Could you check a few things on this model? Use its own coordinates, in mm. Face numbers are marked on the shaded views. A direction names the side the tool comes from. Coordinates: 2 decimals unless noted, no trailing zeros. Order: outer loops, then holes, each group sorted by start corner. A loop starts at its lowest first (then second) coordinate and runs counter-clockwise, first axis right, second up. Notation, with made-up numbers: (76, -31.5) -> (123, -31.5) arc R17 cw to (123, 0.5) -> close; hole circle Ø6 at (-9.75, -40). An arc over 180 degrees is marked (long way). Put each result on its own line as item: value. Start each with the question number.
Q1. For the marked faces 1 and 2, which set-ups out of +Z, -Z, +X, -X, +Y, -Y let a thin tool reach every point of the face, with its end or its side?
Q2. If we section it at A-A (z = 0): Please give me the cut outline in (x, y), and give its area (3 significant figures).
Q3. Please list where these lines run through material, in increasing order: line 1 along X through (y, z) = (3.75, 0); line 2 along Z through (x, y) = (0, 10).
Q4. We'd pull the mould along X, two halves only. Please class the marked faces 3, 4 and 5: +X half, -X half, draft (parallel to the pull), parting line (faces both ways), or undercut.
Q5. If we section it at B-B (y = 9.75): Please give me the cut outline in (x, z).
Q6. Will these pins go through, and if not, where does the flat tip stop? pin 1 (3 mm diameter, centred on y = 6, z = -3, fed in from +X); pin 2 (2 mm diameter, centred on x = -2.5, y = 10.5, fed in from -Z); pin 3 (5 mm diameter, centred on y = 11, z = -1, fed in from +X).
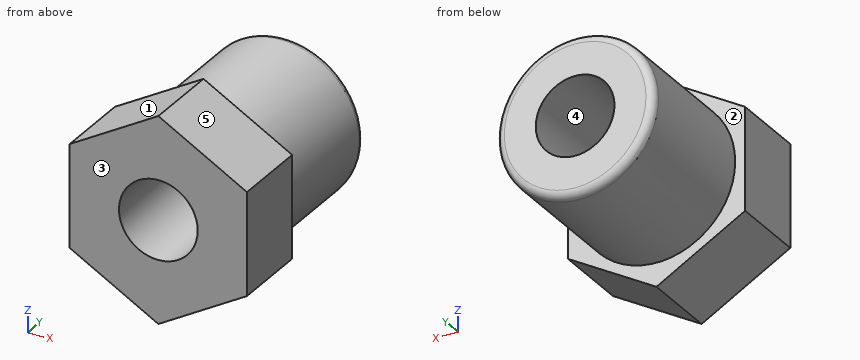
Autodesk Inventor part; units mm, degrees
ref_plane "YZ Plane" through (0, 0, 0) normal (1, 0, 0) x (0, 1, 0)
ref_plane "XZ Plane" through (0, 0, 0) normal (0, 1, 0) x (-1, 0, 0)
ref_plane "XY Plane" through (0, 0, 0) normal (0, 0, 1) x (1, 0, 0)
sketch "Sketch1" plane through (0, 0, 0) normal (0, 1, 0) x (-1, 0, 0)
  line L0 (0, 0) -> (0, -6.5) construction
  line L1 (0, -6.5) -> (0, 6.5) construction
  line L2 (0, -6.5) -> (-5.6292, -3.25)
  line L3 (-5.6292, -3.25) -> (-5.6292, 3.25)
  line L4 (-5.6292, 3.25) -> (0, 6.5)
  line L5 (0, 6.5) -> (5.6292, 3.25)
  line L6 (5.6292, 3.25) -> (5.6292, -3.25)
  line L7 (5.6292, -3.25) -> (0, -6.5)
extrude "Extrusion1" add sketch "Sketch1" along normal blind 5
sketch "Sketch2" plane through (0, 5, 0) normal (0, 1, 0) x (1, 0, 0)
  circle A0 centre (0, 0) radius 2.5
  circle A1 centre (0, 0) radius 5
  dimension "d4" = 5
  dimension "d5" = 10
extrude "Extrusion2" add sketch "Sketch2" along normal blind 9
sketch "Sketch3" plane through (0, 5, 0) normal (0, 1, 0) x (1, 0, 0)
  circle A0 centre (0, 0) radius 2.5
extrude "Extrusion3" cut sketch "Sketch3" against normal through all
thread "Thread1"
fillet "Fillet1" radius 0.5 1 edges at (-5, 14, 0)
properties part number "Premistoppa M10x1"
The answers:
1. face 1: +Z, -X, +Y, -Y
1. face 2: +Y
2. outline: (-5.63, 0) -> (-2.5, 0) -> (-2.5, 14) -> (-4.5, 14) arc R0.5 ccw to (-5, 13.5) -> (-5, 5) -> (-5.63, 5) -> close; (2.5, 0) -> (5.63, 0) -> (5.63, 5) -> (5, 5) -> (5, 13.5) arc R0.5 ccw to (4.5, 14) -> (2.5, 14) -> close
2. area: 76.2 mm^2
3. line 1: -5.63 to -2.5, 2.5 to 5.63
3. line 2: -5 to -2.5, 2.5 to 5
4. face 3: draft
4. face 4: undercut
4. face 5: +X half
5. outline: circle Ø10 at (0, 0); hole circle Ø5 at (0, 0)
6. pin 1: x = 5.63
6. pin 2: z = -4.77
6. pin 3: x = 5
